from build123d import *

# Parameters (mm, degrees)
SKETCH1_W           = 12
SKETCH1_H           = 7
BOSS_EXTRUDE1_DEPTH = 16
CUT_EXTRUDE1_DEPTH  = 20
CUT_EXTRUDE2_REACH  = 20.466
SKETCH3_R           = 2.9
CUT_EXTRUDE3_DEPTH  = 4
SKETCH5_W           = 14
SKETCH5_H           = 40
BOSS_EXTRUDE2_DEPTH = 2.5
CUT_EXTRUDE4_REACH  = 46.623
CUT_EXTRUDE6_DEPTH  = 1.9
CUT_EXTRUDE7_REACH  = 43.251
SKETCH9_R           = 2.9


with BuildPart() as part:
    # Sketch1 → Boss-Extrude1 (new body)
    with BuildSketch(Plane(origin=(0, 0, 0), x_dir=(1, 0, 0), z_dir=(0, 1, 0))):
        Rectangle(SKETCH1_W, SKETCH1_H)
    extrude(amount=BOSS_EXTRUDE1_DEPTH)

    # Sketch2 → Cut-Extrude1 (cut)
    with BuildSketch(Plane(origin=(0, 16, 0), x_dir=(1, 0, 0), z_dir=(0, 1, 0))):
        Polygon((0, 3.5), (2.25, 3.5), (4.25, 1.5), (0, 1.5), (-4.25, 1.5), (-2.25, 3.5), align=None)
    extrude(amount=-CUT_EXTRUDE1_DEPTH, mode=Mode.SUBTRACT)

    # Sketch3 → Cut-Extrude2 (cut, up to next)
    with BuildSketch(Plane.XY.offset(3.5), mode=Mode.PRIVATE) as cut_extrude2_sk1:
        with Locations((0, 7.35)):
            Circle(SKETCH3_R)
    cut_extrude2_tool1 = extrude(cut_extrude2_sk1.sketch, amount=-CUT_EXTRUDE2_REACH, mode=Mode.PRIVATE) & part.part
    add(cut_extrude2_tool1.solids().sort_by_distance((0, 7.35, 3.5))[0], mode=Mode.SUBTRACT)

    # Sketch4 → Cut-Extrude3 (cut)
    with BuildSketch(Plane.XY.offset(3.5)):
        Polygon((0, 13.700852961), (-5.5, 10.525426481), (-5.5, 4.174573519), (0, 0.999147039), (5.5, 4.174573519), (5.5, 10.525426481), align=None)
    extrude(amount=-CUT_EXTRUDE3_DEPTH, mode=Mode.SUBTRACT)

    # Sketch5 → Boss-Extrude2 (add)
    with BuildSketch(Plane(origin=(0, 16, 0), x_dir=(1, 0, 0), z_dir=(0, 1, 0))):
        with Locations((0, -16.5)):
            Rectangle(SKETCH5_W, SKETCH5_H)
    extrude(amount=BOSS_EXTRUDE2_DEPTH)

    # Sketch6 → Cut-Extrude4 (cut, up to next)
    with BuildSketch(Plane(origin=(0, 0, -3.5), x_dir=(-1, 0, 0), z_dir=(0, 0, -1)), mode=Mode.PRIVATE) as cut_extrude4_sk1:
        Polygon((-7, 16), (-7, 18.5), (-6, 16), align=None)
    cut_extrude4_tool1 = extrude(cut_extrude4_sk1.sketch, amount=-CUT_EXTRUDE4_REACH, mode=Mode.PRIVATE) & part.part
    # Sketch6 → Cut-Extrude4 (cut, up to next)
    with BuildSketch(Plane(origin=(0, 0, -3.5), x_dir=(-1, 0, 0), z_dir=(0, 0, -1)), mode=Mode.PRIVATE) as cut_extrude4_sk2:
        Polygon((7, 16), (6, 16), (7, 18.5), align=None)
    cut_extrude4_tool2 = extrude(cut_extrude4_sk2.sketch, amount=-CUT_EXTRUDE4_REACH, mode=Mode.PRIVATE) & part.part
    add(cut_extrude4_tool1.solids().sort_by_distance((6.666667, 16.833333, -3.5))[0], mode=Mode.SUBTRACT)
    add(cut_extrude4_tool2.solids().sort_by_distance((-6.666667, 16.833333, -3.5))[0], mode=Mode.SUBTRACT)

    # Sketch8 → Cut-Extrude6 (cut)
    with BuildSketch(Plane.XZ.offset(-16)):
        Polygon((0, 22.599147039), (5.5, 25.774573519), (5.5, 32.125426481), (0, 35.300852961), (-5.5, 32.125426481), (-5.5, 25.774573519), align=None)
    extrude(amount=-CUT_EXTRUDE6_DEPTH, mode=Mode.SUBTRACT)

    # Sketch9 → Cut-Extrude7 (cut, up to next)
    with BuildSketch(Plane(origin=(0, 17.9, 0), x_dir=(-1, 0, 0), z_dir=(0, -1, 0)), mode=Mode.PRIVATE) as cut_extrude7_sk1:
        with Locations(Location((0, -28.95, 0), (0, 0, 90))):
            Circle(SKETCH9_R)
    cut_extrude7_tool1 = extrude(cut_extrude7_sk1.sketch, amount=-CUT_EXTRUDE7_REACH, mode=Mode.PRIVATE) & part.part
    add(cut_extrude7_tool1.solids().sort_by_distance((0, 17.9, 28.95))[0], mode=Mode.SUBTRACT)


solid = part.part
Read the model definition and answer for the solid it produces. Units are mm, in the model's axes. A direction names the side the tool comes from. Round coordinates to 2 decimals unless told otherwise and drop trailing zeros. Write each loop counter-clockwise with the first axis right and the second up, starting at its lowest first coordinate (ties: lowest second). Pieces come first, ordered by that corner, then holes. Notation, with made-up numbers: (77, -40) - (124, -40) arc R16 cw to (124, -28) - close; hole circle Ø11 at (27, -37). An arc over 180 degrees is marked (long way). One line per question, with ' | ' between items. Start each with the question number.
1. Each of these flat-tipped pins is pushed along its axis until it touches: pin 1 (0.6 mm diameter, centred on y = 17, z = 29.5, fed in from -X); pin 2 (5 mm diameter, centred on x = -5, y = 6.5, fed in from +Z); pin 3 (5 mm diameter, centred on x = 0, z = 28.95, fed in from -Y); pin 4 (6 mm diameter, centred on y = 15, z = 10.5, fed in from +X). Where does it stop, or does it pass through?
2. Find the intervals of material crossed by probe 1 along Y at (x, z) = (0, -0.85); probe 2 along Z at (x, y) = (3.5, 1.5); probe 3 along Z at (x, y) = (3.5, 9.5), in increasing order. Write a range as [from, to].
3. Section A-A (y = 17) is taken. Determine the outline of the cut face in (x, z), and give its area (3 significant figures).
4. For a pull along X with two mould halves and no side action, classify faces 4 (the face through (0, 18.5, 16)), 5 (the face through (-6, 8, 0)), 6 (the face through (0.128, 18.196, 31.847)) as +X half, -X half, draft (parallel to the pull), parting line (faces both ways), or undercut.
5. Section C-C (x = -1) is taken. Determine the outline of the cut face in (y, z), and give its area (3 significant figures).
6. Section B-B (z = 28.95) is taken. Determine the outline of the cut face in (x, y).
7. For faces 1 (the face through (-2.79, 2.61, 1.53)), 2 (the face through (2.712, 16.937, 24.165)), 3 (the face through (0, 16, 16)), determine the directions among +Z, -Z, +X, -X, +Y, -Y from which every point of the face is accessible in a straight line to the end or side of a thin tool.
8. Section D-D (y = 7.35) is taken. Determine the outline of the cut face in (x, z).
Filled in:
1) pin 1: x = -6.52 | pin 2: z = 3.5 | pin 3: through | pin 4: x = 6.8
2) probe 1: [0, 4.45], [10.25, 18.5] | probe 2: [-3.5, -2.25], [-1.5, 3.5] | probe 3: [-3.5, -2.25], [-1.5, -0.5]
3) outline: (-6.4, -3.5) - (6.4, -3.5) - (6.4, 36.5) - (-6.4, 36.5) - close; hole (-5.5, 25.77) - (0, 22.6) - (5.5, 25.77) - (5.5, 32.13) - (0, 35.3) - (-5.5, 32.13) - close | area: 407 mm²
4) face 4: draft | face 5: -X half | face 6: undercut
5) outline: (0, -1.5) - (4.63, -1.5) - (4.63, -0.5) - (1.58, -0.5) - (1.58, 3.5) - (0, 3.5) - close; (10.07, -1.5) - (16, -1.5) - (16, -3.5) - (18.5, -3.5) - (18.5, 26.23) - (17.9, 26.23) - (17.9, 23.18) - (16, 23.18) - (16, 3.5) - (13.12, 3.5) - (13.12, -0.5) - (10.07, -0.5) - close; (16, 34.72) - (17.9, 34.72) - (17.9, 31.67) - (18.5, 31.67) - (18.5, 36.5) - (16, 36.5) - close | area: 103 mm²
6) outline: (-7, 18.5) - (-6, 16) - (-5.5, 16) - (-5.5, 17.9) - (-2.9, 17.9) - (-2.9, 18.5) - close; (2.9, 17.9) - (5.5, 17.9) - (5.5, 16) - (6, 16) - (7, 18.5) - (2.9, 18.5) - close
7) face 1: +Z | face 2: -Y | face 3: +Z, +X, -X, -Y
8) outline: (-6, -3.5) - (-2.25, -3.5) - (-4.25, -1.5) - (-2.9, -1.5) - (-2.9, -0.5) - (-5.5, -0.5) - (-5.5, 3.5) - (-6, 3.5) - close; (2.25, -3.5) - (6, -3.5) - (6, 3.5) - (5.5, 3.5) - (5.5, -0.5) - (2.9, -0.5) - (2.9, -1.5) - (4.25, -1.5) - close
